```python
from build123d import *

# Parameters (mm, degrees)
F0_W     = 16
F0_H     = 12
F1_DEPTH = 1.75
F2_W     = 10.5
F2_H     = 10.5
F3_DEPTH = 3
F4_R     = 0.25
F5_DEPTH = 5


with BuildPart() as f1:
    # F0 (on Top) → F1 (new body)
    with BuildSketch(Plane.XY):
        Rectangle(F0_W, F0_H)
    extrude(amount=F1_DEPTH)

    # F2 (on face) → F3 (join)
    with BuildSketch(Plane.XY.offset(1.75)):
        Rectangle(F2_W, F2_H)
    extrude(amount=F3_DEPTH)

    # F4 (on face) → F5 (join)
    with BuildSketch(Plane(origin=(0, 0, 0), x_dir=(1, 0, 0), z_dir=(0, 0, -1))):
        with Locations((-6.25, 0)):
            Circle(F4_R)
        with Locations((6.25, 0)):
            Circle(F4_R)
    extrude(amount=F5_DEPTH)


solid = f1.part
```
Part model, mm, in its own coordinate system. A direction names the side the tool comes from. Coordinates: 2 decimals unless noted, no trailing zeros. Write each loop counter-clockwise with the first axis right and the second up, starting at its lowest first coordinate (ties: lowest second). Pieces come first, ordered by that corner, then holes.
Item 1: Slice it at A-A (x = -0.5). Write the cut outline in (y, z).
Item 2: Pin check, flat tips, straight feed: pin 1 (2.5 mm diameter, centred on y = -2, z = 4, fed in from -X); pin 2 (3 mm diameter, centred on x = 2.5, y = -4, fed in from -Z); pin 3 (2.5 mm diameter, centred on x = 2, z = 3.5, fed in from -Y). Stop position of each tip, or through.
Item 3: Slice it at D-D (z = 2.25). Write the cut outline in (x, y).
Item 4: Probe line 1 (Z direction, x = 2.75, y = -0.25); line 2 (X direction, y = -2.5, z = 4). List the from-to ranges inside material, lowest first.
Item 5: Slice it at C-C (z = -3). Write the cut outline in (x, y).
Item 6: Slice it at B-B (y = -2). Write the cut outline in (x, z), and give its area (3 significant figures).
Item 7: Which spindle directions (+Z, -Z, +X, -X, +Y, -Y) get a long thin tool onto all of the face, cutting with end or side? Do faces 1 (the face through (0, 5.25, 3)), 2 (the face through (0, -5.25, 3)), 3 (the face through (-5.25, 0, 3)). Say none if no direction does.
Results found:
1. outline: (-6, 0) - (6, 0) - (6, 1.75) - (5.25, 1.75) - (5.25, 4.75) - (-5.25, 4.75) - (-5.25, 1.75) - (-6, 1.75) - close
2. pin 1: stops at x = -5.25
2. pin 2: stops at z = 0
2. pin 3: stops at y = -5.25
3. outline: (-5.25, -5.25) - (5.25, -5.25) - (5.25, 5.25) - (-5.25, 5.25) - close
4. line 1: z = 0 to 4.75
4. line 2: x = -5.25 to 5.25
5. outline: circle Ø0.5 at (-6.25, 0); circle Ø0.5 at (6.25, 0)
6. outline: (-8, 0) - (8, 0) - (8, 1.75) - (5.25, 1.75) - (5.25, 4.75) - (-5.25, 4.75) - (-5.25, 1.75) - (-8, 1.75) - close
6. area: 59.5 mm2
7. face 1: +Z, +X, -X, +Y
7. face 2: +Z, +X, -X, -Y
7. face 3: +Z, -X, +Y, -Y
